Autodesk Inventor part; units mm, degrees
ref_plane "YZ Plane" through (0, 0, 0) normal (1, 0, 0) x (0, 1, 0)
ref_plane "XZ Plane" through (0, 0, 0) normal (0, 1, 0) x (-1, 0, 0)
ref_plane "XY Plane" through (0, 0, 0) normal (0, 0, 1) x (1, 0, 0)
sketch "Sketch1" plane through (0, 0, 0) normal (0, 1, 0) x (-1, 0, 0)
  circle A0 centre (0, 0) radius 6.35
  line L0 (0, -9.2376) -> (-8, -4.6188)
  line L1 (-8, -4.6188) -> (-8, 4.6188)
  line L2 (-8, 4.6188) -> (0, 9.2376)
  line L3 (0, 9.2376) -> (8, 4.6188)
  line L4 (8, 4.6188) -> (8, -4.6188)
  line L5 (8, -4.6188) -> (0, -9.2376)
  dimension "d0" = 12.7
  dimension "d3" = 16
extrude "Extrusion1" add sketch "Sketch1" along normal mid plane 1071.516 contours A0 | L0 L1 L2 L3 L4 L5
sketch "Sketch2" plane through (0, 535.758, 0) normal (0, 1, 0) x (1, 0, 0)
  point P0 (0, 0)
  point P1 (0, 0)
hole "Hole1" at (0, 535.758, 0) direction (0, -1, 0) diameter 4.917 depth 10
sketch "Sketch3" plane through (0, -535.758, 0) normal (0, -1, 0) x (1, 0, 0)
  point P0 (0, 0)
  point P1 (0, 0)
hole "Hole2" at (0, -535.758, 0) direction (0, 1, 0) diameter 4.917 depth 10
properties part number "SP17V1 Varilla Pedal"
Could you check a few things on this model? Use its own coordinates, in mm. Coordinates: 2 decimals unless noted, no trailing zeros. Order: outer loops, then holes, each group sorted by start corner. A loop starts at its lowest first (then second) coordinate and runs counter-clockwise, first axis right, second up. Notation, with made-up numbers: (-38.5, 42.25) - (14.5, 42.25) arc R19 cw to (14.5, 66.25) - close; hole circle Ø11 at (0, -1.75). An arc over 180 degrees is marked (long way). Answer in a Markdown table with one row per item. Add a question column.
(1) I need wall thicknesses on L1, parallel to X at y = -529, z = 0; L2, parallel to Z at x = 0, y = -527.75; L3, parallel to Z at x = 2, y = -198. Which ranges of each line are inside material? Lowest first, please.
(2) If we section it at A-A, the plane y = -25.5: Please give me the cut outline in (x, z).
(3) If we section it at B-B, the plane x = -5: Please give me the cut outline in (y, z), then the cut area to 3 significant figures.
(4) Will these pins go through, and if not, where does the flat tip stop? pin 1 (5.5 mm diameter, centred on x = 0, z = 0, fed in from +Y); pin 2 (4.5 mm diameter, centred on x = 0, z = 0, fed in from -Y); pin 3 (1.5 mm diameter, centred on x = 4, y = 78.5, fed in from -Z); pin 4 (2 mm diameter, centred on x = -6, y = 314.5, fed in from +Z).
Results are:
| question | item | result |
|---|---|---|
| 1 | L1 | x = -8 to -2.46, 2.46 to 8 |
| 1 | L2 | z = -9.24 to -2.46, 2.46 to 9.24 |
| 1 | L3 | z = -8.08 to 8.08 |
| 2 | outline | (-8, -4.62) - (0, -9.24) - (8, -4.62) - (8, 4.62) - (0, 9.24) - (-8, 4.62) - close |
| 3 | outline | (-535.76, -6.35) - (535.76, -6.35) - (535.76, 6.35) - (-535.76, 6.35) - close |
| 3 | area | 13,600 mm2 |
| 4 | pin 1 | stops at y = 535.76 |
| 4 | pin 2 | stops at y = -525.76 |
| 4 | pin 3 | stops at z = -7.36 |
| 4 | pin 4 | stops at z = 6.35 |
